```python
from build123d import *

# Parameters (mm, degrees)
SKETCH1_W           = 60
SKETCH1_H           = 93
BOSS_EXTRUDE1_DEPTH = 15
SKETCH2_W           = 37
SKETCH2_H           = 37
BOSS_EXTRUDE2_DEPTH = 15


with BuildPart() as part:
    # Sketch1 → Boss-Extrude1 (new body)
    with BuildSketch(Plane(origin=(0, 0, 0), x_dir=(0, 1, 0), z_dir=(0, 0, 1))):
        Rectangle(SKETCH1_W, SKETCH1_H)
    extrude(amount=BOSS_EXTRUDE1_DEPTH)

    # Sketch2 → Boss-Extrude2 (add)
    with BuildSketch(Plane.XY.offset(15)):
        Rectangle(SKETCH2_W, SKETCH2_H)
    extrude(amount=BOSS_EXTRUDE2_DEPTH)


solid = part.part
```
Here's how the part is built. I have some questions about the finished solid (model axes, mm). A direction names the side the tool comes from. Give positions to 0.01 mm unless a question says otherwise; leave off trailing zeros. Order: outer loops, then holes, each group sorted by start corner. A loop starts at its lowest first (then second) coordinate and runs counter-clockwise, first axis right, second up. Notation, with made-up numbers: (-18.75, 30) - (29.25, 30) arc R10 ccw to (29.25, 47) - close; hole circle Ø5 at (51, 41). An arc over 180 degrees is marked (long way). Answer as a JSON object with one key per item and string values. Group by question number.
Item 1: If we section it at B-B on x = 14.5: Please give me the cut outline in (y, z).
Item 2: Please list where these lines run through material, in increasing order: probe 1 along Z at (x, y) = (41, 1); probe 2 along X at (y, z) = (7.5, 21.75).
Item 3: Which directions (+Z, -Z, +X, -X, +Y, -Y) give clear straight access to the entire face, cutting with the end or side of a thin tool? Please do faces 1 (the flat face through (-18.5, 0, 22)), 2 (the flat face through (0, -18.5, 22)), 3 (the flat face through (0, 18.5, 22)), 4 (the flat face through (18.5, 0, 22)).
Item 4: For P1, Ø5, axis at x = 21.5, y = 14.5, coming from the +Z side; P2, Ø4.5, axis at x = -4.5, z = 19, coming from the -Y side, each with a flat end and sliding along its axis, tell me the tip position at first contact or that it passes through.
Item 5: If we section it at A-A on y = -5: Please give me the cut outline in (x, z).
Item 6: If we section it at D-D on y = -21.5: Please give me the cut outline in (x, z), and give its area (4 significant figures).
Item 7: If we section it at C-C on z = 24.75: Please give me the cut outline in (x, y).
Result set:
{
 "1": {"outline": "(-30, 0) - (30, 0) - (30, 15) - (18.5, 15) - (18.5, 30) - (-18.5, 30) - (-18.5, 15) - (-30, 15) - close"},
 "2": {"probe 1": "0 to 15", "probe 2": "-18.5 to 18.5"},
 "3": {"face 1": "+Z, -X, +Y, -Y", "face 2": "+Z, +X, -X, -Y", "face 3": "+Z, +X, -X, +Y", "face 4": "+Z, +X, +Y, -Y"},
 "4": {"P1": "z = 15", "P2": "y = -18.5"},
 "5": {"outline": "(-46.5, 0) - (46.5, 0) - (46.5, 15) - (18.5, 15) - (18.5, 30) - (-18.5, 30) - (-18.5, 15) - (-46.5, 15) - close"},
 "6": {"outline": "(-46.5, 0) - (46.5, 0) - (46.5, 15) - (-46.5, 15) - close", "area": "1,395 mm²"},
 "7": {"outline": "(-18.5, -18.5) - (18.5, -18.5) - (18.5, 18.5) - (-18.5, 18.5) - close"}
}
